The listing builds one solid part. Answer for the finished solid, in the listing's coordinates (mm). Give positions to 0.01 mm unless a question says otherwise; leave off trailing zeros. Order: outer loops, then holes, each group sorted by start corner. A loop starts at its lowest first (then second) coordinate and runs counter-clockwise, first axis right, second up. Notation, with made-up numbers: (-25.5, 5.25) - (-16.5, 5.25) arc R32 cw to (-16.5, 38.25) - close; hole circle Ø1 at (-0.5, 45). An arc over 180 degrees is marked (long way). Answer in a Markdown table with one row per item.
from build123d import *

# Parameters (mm, degrees)
SKETCH1_W            = 1.778
SKETCH1_H            = 6.858
BOSS_EXTRUDE1_DEPTH  = 4.318
SKETCH3_R            = 0.254
CUT_EXTRUDE2_DEPTH   = 6.585112891
LPATTERN2_COUNT      = 10
LPATTERN2_PITCH      = 0.65
LPATTERN2_COUNT_DIR2 = 2
LPATTERN2_PITCH_DIR2 = 0.77


with BuildPart() as part:
    # Sketch1 → Boss-Extrude1 (new body)
    with BuildSketch(Plane(origin=(0, 0, 0), x_dir=(1, 0, 0), z_dir=(0, 1, 0))):
        Rectangle(SKETCH1_W, SKETCH1_H)
    extrude(amount=BOSS_EXTRUDE1_DEPTH)

    # Sketch3 → Cut-Extrude2 (cut, through all)
    with BuildSketch(Plane(origin=(0, 4.318, 0), x_dir=(1, 0, 0), z_dir=(0, 1, 0))):
        with Locations(Location((-0.381, -2.921, 0), (0, 0, 270))):
            Circle(SKETCH3_R)
    cut_extrude2 = extrude(amount=-CUT_EXTRUDE2_DEPTH, mode=Mode.SUBTRACT)

    # LPattern2: Cut-Extrude2 10 × 2
    with Locations(*[(j * LPATTERN2_PITCH_DIR2, 0, -i * LPATTERN2_PITCH) for i in range(LPATTERN2_COUNT) for j in range(LPATTERN2_COUNT_DIR2) if (i, j) != (0, 0)]):
        add(cut_extrude2, mode=Mode.SUBTRACT)


solid = part.part
Item 1: Find section A-A on z = 2.25. Write down the section's boundary in (x, y).
Answer block:
| item | result |
|---|---|
| outline | (-0.89, 0) - (-0.63, 0) - (-0.63, 4.32) - (-0.89, 4.32) - close; (-0.13, 0) - (0.14, 0) - (0.14, 4.32) - (-0.13, 4.32) - close; (0.64, 0) - (0.89, 0) - (0.89, 4.32) - (0.64, 4.32) - close |
Item 2: Find section B-B on y = 0.75. Count the separate pieces of the cut face and the enclosed holes in it, then the cut area to 3 significant figures.
Answer block:
| item | result |
|---|---|
| separate pieces | 1 |
| enclosed holes | 20 |
| area | 8.14 mm² |
Item 3: Consider line 1 (X direction, y = 1.45, z = 1); line 2 (X direction, y = 1.9, z = -1.75). Determine where each line is inside the solid, lowest interval first.
Answer block:
| item | result |
|---|---|
| line 1 | -0.89 to -0.63, -0.13 to 0.14, 0.64 to 0.89 |
| line 2 | -0.89 to -0.6, -0.16 to 0.17, 0.61 to 0.89 |
Item 4: Find section C-C on z = -1.75. Write down the section's boundary in (x, y).
Answer block:
| item | result |
|---|---|
| outline | (-0.89, 0) - (-0.6, 0) - (-0.6, 4.32) - (-0.89, 4.32) - close; (-0.16, 0) - (0.17, 0) - (0.17, 4.32) - (-0.16, 4.32) - close; (0.61, 0) - (0.89, 0) - (0.89, 4.32) - (0.61, 4.32) - close |
